Autodesk Inventor part; units mm, degrees
ref_plane "Work Plane1" through (-18.1, 0, 3.4982) normal (0, 0, 1) x (1, 0, 0)
ref_plane "Work Plane2" through (0, -10.5, -7.5) normal (0, 0, 1) x (1, 0, 0)
ref_plane "YZ Plane" through (0, 0, 0) normal (1, 0, 0) x (0, 1, 0)
sketch "Sketch1" plane through (0, 0, 0) normal (0, 0, 1) x (1, 0, 0)
  circle A0 centre (0, 0) radius 4
  circle A1 centre (-18.1, 0) radius 2.9 construction
  circle A2 centre (29.9, -108.4) radius 1.6
  circle A3 centre (-66.1, -108.4) radius 1.6
  circle A4 centre (-66.1, 17.4) radius 1.6
  circle A5 centre (29.9, 17.4) radius 1.6
  line L0 (29.9, 17.4) -> (-66.1, 17.4) construction
  line L1 (37.9, -116.4) -> (-74.1, -116.4)
  line L2 (-74.1, -116.4) -> (-74.1, 25.4)
  line L3 (-74.1, 25.4) -> (37.9, 25.4)
  line L4 (37.9, 25.4) -> (37.9, -116.4)
  line L5 (-66.1, -108.4) -> (-66.1, 17.4) construction
  circle A6 centre (-18.1, 0) radius 4
  point P0 (-18.1, 17.4)
  point P1 (-18.1, 25.4)
  point P2 (-66.1, -45.5)
  point P3 (-74.1, -45.5)
  dimension "d0" = 3.2
  dimension "d1" = 96
  dimension "d2" = 125.8
  dimension "d3" = 141.8
  dimension "d4" = 112
  dimension "d5" = 25.4
  dimension "d11" = 8
ref_plane "Work Plane1" through (-18.1, 0, 3.4982) normal (0, 0, 1) x (1, 0, 0)
extrude "Extrusion1" add sketch "Sketch1" along normal blind 4
chamfer "Chamfer1" distance 5 distance2 2 1 edges at (-4, 0, 4) measured on face at (-17.9393, -72.8829, 4)
fillet "Fillet1" radius 8 4 edges at (37.9, 25.4, 2) (-74.1, 25.4, 2) (-74.1, -116.4, 2) (37.9, -116.4, 2)
sketch "Sketch2" plane through (0, 0, 4) normal (0, 0, 1) x (1, 0, 0)
  line L0 (32.7, -97.35) -> (-68.9, -97.35) construction
  line L1 (-68.9, -97.35) -> (-68.9, 4.25) construction
  line L2 (-68.9, 4.25) -> (32.7, 4.25) construction
  line L3 (32.7, 4.25) -> (32.7, -97.35) construction
  line L4 (-66.1, -116.4) -> (29.9, -116.4) construction
  point P0 (0, 0)
  point P1 (-18.1, -116.4)
  point P2 (-18.1, -97.35)
  dimension "d25" = 101.6
  dimension "d31" = 19.05
fillet "Fillet2" radius 2 1 edges at (-22.1, 0, 0)
sketch "Sketch3" plane through (0, 0, 0) normal (0, 0, -1) x (-1, 0, 0)
  circle A0 centre (43.1, -6) radius 1 construction
  circle A1 centre (-8.9, 5) radius 1 construction
  circle A2 centre (43.1, -6) radius 0.75
  circle A3 centre (-8.9, 5) radius 0.75
  circle A4 centre (43.1, -6) radius 1.9
  circle A5 centre (-8.9, 5) radius 1.9
  point P0 (0, 0)
  dimension "d33" = 1.5
  dimension "d34" = 3.8
ref_plane "Work Plane2" through (0, -10.5, -7.5) normal (0, 0, 1) x (1, 0, 0)
extrude "Extrusion2" add sketch "Sketch3" along normal up to surface (7.5 mm away)
fillet "Fillet3" radius 2 2 edges at (-41.2, -6, 0) (10.8, 5, 0)
fillet "Fillet4" radius 3 8 edges at (35.5569, 23.0569, 4) (-18.1, 25.4, 4) (-71.7569, 23.0569, 4) (-74.1, -45.5, 4) (-71.7569, -114.0569, 4) (-18.1, -116.4, 4) (35.5569, -114.0569, 4) (37.9, -45.5, 4)
properties part number "Lid"
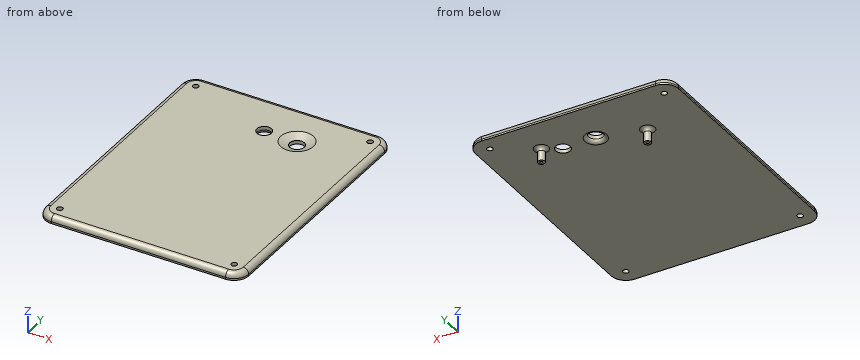
Check sheet for the modelled part. Datum: model origin and axes. Units: mm. Give positions to 0.01 mm unless a question says otherwise; leave off trailing zeros. Order: outer loops, then holes, each group sorted by start corner. A loop starts at its lowest first (then second) coordinate and runs counter-clockwise, first axis right, second up. Notation, with made-up numbers: M -16.5,38 L -5.5,38 A33 cw -5.5,77 Z; hole C 65,0 d8. An arc over 180 degrees is marked long. Answer in a Markdown table with one row per item.
1) Cross-section at B-B, the plane z = -4.5. Enter the section's corners in (x, y).
Filled sheet:
| item | result |
|---|---|
| outline | C -43.1,-6 d3.8; C 8.9,5 d3.8; hole C -43.1,-6 d1.5; hole C 8.9,5 d1.5 |
2) Gauge pin test, flat ends, axial feed: P1, Ø3, axis at x = -66.1, y = -108.4, coming from the +Z side; P2, Ø5, axis at x = 29.9, y = -108.4, coming from the -Z side; P3, Ø1.6, axis at x = 9, y = 5.5, coming from the -Z side. Record the tip position at first contact, or that the pin passes through.
Filled sheet:
| item | result |
|---|---|
| P1 | passes through |
| P2 | stops at z = 0 |
| P3 | stops at z = -7.5 |
3) Thickness scan on L1, parallel to X at y = -108.4, z = 1.45; L2, parallel to Y at x = 8.9, z = -4; L3, parallel to Y at x = 0, z = 1.3. Record the ranges inside material, lowest first. Write a range as [from, to].
Filled sheet:
| item | result |
|---|---|
| L1 | x = [-74.07, -67.7], [-64.5, 28.3], [31.5, 37.87] |
| L2 | y = [3.1, 4.25], [5.75, 6.9] |
| L3 | y = [-116.38, -4], [4, 25.38] |
4) Cross-section at C-C, the plane y = -13. Enter the section's corners in (x, z).
Filled sheet:
| item | result |
|---|---|
| outline | M -74.1,0 L 37.9,0 L 37.9,1 A3 ccw 34.9,4 L -71.1,4 A3 ccw -74.1,1 Z |
5) Cross-section at A-A, the plane x = -18.1. Enter the section's corners in (y, z).
Filled sheet:
| item | result |
|---|---|
| outline | M -116.4,0 L -6,0 A2 ccw -4,2 L -4,4 L -113.4,4 A3 ccw -116.4,1 Z; M 4,2 A2 ccw 6,0 L 25.4,0 L 25.4,1 A3 ccw 22.4,4 L 4,4 Z |
6) Cross-section at D-D, the plane x = -49.5. Enter the section's corners in (y, z), plus the area to 3 significant figures.
Filled sheet:
| item | result |
|---|---|
| outline | M -116.4,0 L 25.4,0 L 25.4,1 A3 ccw 22.4,4 L -113.4,4 A3 ccw -116.4,1 Z |
| area | 563 mm2 |
